from build123d import *

# Parameters (mm, degrees)
F1_DEPTH = 6.35
F2_DEPTH = 6.35
F3_DEPTH = 6.35
F4_DEPTH = 6.35
F5_DEPTH = 6.35


# Not quite as in the source:
# - a feature names something its author has since deleted; it is built from what else it names


with BuildPart() as f1:
    # F0 (on Front) → F1 (new body)
    with BuildSketch(Plane.XZ):
        with BuildLine():
            ThreePointArc((63.0566746496, -7.490379305), (63.3890717721, -3.751743578), (63.5, 0))
            ThreePointArc((63.5, 0), (62.9393473013, 8.4195345051), (61.2672894084, 16.6903939003))
            ThreePointArc((61.2672894084, 16.6903939003), (58.3327446269, 25.0906537239), (54.2527974979, 32.9982418266))
            ThreePointArc((54.2527974979, 32.9982418266), (47.291532101, 42.3764202304), (38.730412603, 50.3210208521))
            ThreePointArc((38.730412603, 50.3210208521), (29.9555685969, 55.9903019284), (20.3699341201, 60.1441250991))
            ThreePointArc((20.3699341201, 60.1441250991), (7.3544916147, 63.0726680353), (-5.9855682874, 63.2172679912))
            ThreePointArc((-5.9855682874, 63.2172679912), (-13.2670335267, 62.09859758), (-20.3699341201, 60.1441250991))
            ThreePointArc((-20.3699341201, 60.1441250991), (-29.9555685969, 55.9903019284), (-38.730412603, 50.3210208521))
            ThreePointArc((-38.730412603, 50.3210208521), (-47.291532101, 42.3764202304), (-54.2527974979, 32.9982418266))
            ThreePointArc((-54.2527974979, 32.9982418266), (-58.3327446269, 25.0906537239), (-61.2672894084, 16.6903939003))
            ThreePointArc((-61.2672894084, 16.6903939003), (-63.3268462658, 4.6862076377), (-63.0566746496, -7.490379305))
            ThreePointArc((-63.0566746496, -7.490379305), (-60.5844983842, -19.0202143924), (-56.023116606, -29.8941533708))
            ThreePointArc((-56.023116606, -29.8941533708), (-49.318773707, -39.9988569841), (-40.8158107072, -48.6448311366))
            ThreePointArc((-40.8158107072, -48.6448311366), (-33.4288158961, -53.9885568226), (-25.3527004473, -58.2193316694))
            ThreePointArc((-25.3527004473, -58.2193316694), (-15.8671551858, -61.4856356095), (-5.9855682874, -63.2172679912))
            ThreePointArc((-5.9855682874, -63.2172679912), (1.1186954333, -63.4901450662), (8.2089360928, -62.9671610304))
            ThreePointArc((8.2089360928, -62.9671610304), (16.9479005402, -61.1965576424), (25.3527004473, -58.2193316694))
            ThreePointArc((25.3527004473, -58.2193316694), (33.4288158961, -53.9885568226), (40.8158107072, -48.6448311366))
            ThreePointArc((40.8158107072, -48.6448311366), (49.318773707, -39.9988569841), (56.023116606, -29.8941533708))
            ThreePointArc((56.023116606, -29.8941533708), (60.5844983842, -19.0202143924), (63.0566746496, -7.490379305))
        make_face()
        with BuildLine():
            ThreePointArc((61.2672894084, 16.6903939003), (62.9393473013, 8.4195345051), (63.5, 0))
            ThreePointArc((63.5, 0), (63.3890717721, -3.751743578), (63.0566746496, -7.490379305))
            Line((63.0566746496, -7.490379305), (88.5324627161, 16.6903939003))
            Line((88.5324627161, 16.6903939003), (61.2672894084, 16.6903939003))
        make_face()
        with BuildLine():
            ThreePointArc((54.2527974979, 32.9982418266), (58.3327446269, 25.0906537239), (61.2672894084, 16.6903939003))
            Line((61.2672894084, 16.6903939003), (71.193754673, 45.4481393099))
            Line((71.193754673, 45.4481393099), (54.2527974979, 32.9982418266))
        make_face()
        with BuildLine():
            Line((85.9054028988, -7.490379305), (63.0566746496, -7.490379305))
            ThreePointArc((63.0566746496, -7.490379305), (60.5844983842, -19.0202143924), (56.023116606, -29.8941533708))
            Line((56.023116606, -29.8941533708), (85.9054028988, -7.490379305))
        make_face()
        with BuildLine():
            ThreePointArc((38.730412603, 50.3210208521), (47.291532101, 42.3764202304), (54.2527974979, 32.9982418266))
            Line((54.2527974979, 32.9982418266), (54.2527974979, 61.2032547377))
            Line((54.2527974979, 61.2032547377), (38.730412603, 50.3210208521))
        make_face()
        with BuildLine():
            ThreePointArc((20.3699341201, 60.1441250991), (29.9555685969, 55.9903019284), (38.730412603, 50.3210208521))
            Line((38.730412603, 50.3210208521), (38.0926132202, 72.2317844629))
            Line((38.0926132202, 72.2317844629), (20.3699341201, 60.1441250991))
        make_face()
        with BuildLine():
            Line((60.1600408554, -63.261911273), (40.8158107072, -48.6448311366))
            ThreePointArc((40.8158107072, -48.6448311366), (33.4288158961, -53.9885568226), (25.3527004473, -58.2193316694))
            Line((25.3527004473, -58.2193316694), (60.1600408554, -63.261911273))
        make_face()
        with BuildLine():
            ThreePointArc((-20.3699341201, 60.1441250991), (-13.2670335267, 62.09859758), (-5.9855682874, 63.2172679912))
            Line((-5.9855682874, 63.2172679912), (-20.3699341201, 81.6848352551))
            Line((-20.3699341201, 81.6848352551), (-20.3699341201, 60.1441250991))
        make_face()
        with BuildLine():
            ThreePointArc((-38.730412603, 50.3210208521), (-29.9555685969, 55.9903019284), (-20.3699341201, 60.1441250991))
            Line((-20.3699341201, 60.1441250991), (-38.0926132202, 72.2317844629))
            Line((-38.0926132202, 72.2317844629), (-38.730412603, 50.3210208521))
        make_face()
        with BuildLine():
            ThreePointArc((-54.2527974979, 32.9982418266), (-47.291532101, 42.3764202304), (-38.730412603, 50.3210208521))
            Line((-38.730412603, 50.3210208521), (-54.2527974979, 61.2032547377))
            Line((-54.2527974979, 61.2032547377), (-54.2527974979, 32.9982418266))
        make_face()
        with BuildLine():
            Line((-60.1600408554, -63.261911273), (-25.3527004473, -58.2193316694))
            ThreePointArc((-25.3527004473, -58.2193316694), (-33.4288158961, -53.9885568226), (-40.8158107072, -48.6448311366))
            Line((-40.8158107072, -48.6448311366), (-60.1600408554, -63.261911273))
        make_face()
        with BuildLine():
            ThreePointArc((-61.2672894084, 16.6903939003), (-58.3327446269, 25.0906537239), (-54.2527974979, 32.9982418266))
            Line((-54.2527974979, 32.9982418266), (-71.193754673, 45.4481393099))
            Line((-71.193754673, 45.4481393099), (-61.2672894084, 16.6903939003))
        make_face()
        with BuildLine():
            ThreePointArc((-63.0566746496, -7.490379305), (-63.3268462658, 4.6862076377), (-61.2672894084, 16.6903939003))
            Line((-61.2672894084, 16.6903939003), (-88.5324627161, 16.6903939003))
            Line((-88.5324627161, 16.6903939003), (-63.0566746496, -7.490379305))
        make_face()
        with BuildLine():
            Line((-85.9054028988, -7.490379305), (-56.023116606, -29.8941533708))
            ThreePointArc((-56.023116606, -29.8941533708), (-60.5844983842, -19.0202143924), (-63.0566746496, -7.490379305))
            Line((-63.0566746496, -7.490379305), (-85.9054028988, -7.490379305))
        make_face()
    extrude(amount=F1_DEPTH)

    # F0 (on Front) → F2 (join)
    with BuildSketch(Plane.XZ):
        with BuildLine():
            Line((-73.2954144478, -38.053765893), (-40.8158107072, -48.6448311366))
            ThreePointArc((-40.8158107072, -48.6448311366), (-49.318773707, -39.9988569841), (-56.023116606, -29.8941533708))
            Line((-56.023116606, -29.8941533708), (-73.2954144478, -38.053765893))
        make_face()
        with BuildLine():
            Line((73.2954144478, -38.053765893), (56.023116606, -29.8941533708))
            ThreePointArc((56.023116606, -29.8941533708), (49.318773707, -39.9988569841), (40.8158107072, -48.6448311366))
            Line((40.8158107072, -48.6448311366), (73.2954144478, -38.053765893))
        make_face()
    extrude(amount=F2_DEPTH)

    # F0 (on Front) → F3 (join)
    with BuildSketch(Plane.XZ):
        with BuildLine():
            Line((0, -92.2421216965), (8.2089360928, -62.9671610304))
            ThreePointArc((8.2089360928, -62.9671610304), (1.1186954333, -63.4901450662), (-5.9855682874, -63.2172679912))
            Line((-5.9855682874, -63.2172679912), (0, -92.2421216965))
        make_face()
        with BuildLine():
            ThreePointArc((-5.9855682874, 63.2172679912), (7.3544916147, 63.0726680353), (20.3699341201, 60.1441250991))
            Line((20.3699341201, 60.1441250991), (0, 92.2421216965))
            Line((0, 92.2421216965), (-5.9855682874, 63.2172679912))
        make_face()
    extrude(amount=F3_DEPTH)

    # F0 (on Front) → F4 (join)
    with BuildSketch(Plane.XZ):
        with BuildLine():
            Line((-20.3699341201, -81.6848352551), (-5.9855682874, -63.2172679912))
            ThreePointArc((-5.9855682874, -63.2172679912), (-15.8671551858, -61.4856356095), (-25.3527004473, -58.2193316694))
            Line((-25.3527004473, -58.2193316694), (-20.3699341201, -81.6848352551))
        make_face()
        with BuildLine():
            Line((60.1600408554, -63.261911273), (40.8158107072, -48.6448311366))
            ThreePointArc((40.8158107072, -48.6448311366), (33.4288158961, -53.9885568226), (25.3527004473, -58.2193316694))
            Line((25.3527004473, -58.2193316694), (60.1600408554, -63.261911273))
        make_face()
    extrude(amount=F4_DEPTH)

    # F0 (on Front) → F5 (join)
    with BuildSketch(Plane.XZ):
        with BuildLine():
            Line((22.25664258, -86.1358046532), (25.3527004473, -58.2193316694))
            ThreePointArc((25.3527004473, -58.2193316694), (16.9479005402, -61.1965576424), (8.2089360928, -62.9671610304))
            Line((8.2089360928, -62.9671610304), (22.25664258, -86.1358046532))
        make_face()
    extrude(amount=F5_DEPTH)


solid = f1.part
Geometry check sheet. Reference: the model listing, model coordinates, mm. A direction names the side the tool comes from. Give positions to 0.01 mm unless a question says otherwise; leave off trailing zeros. Order: outer loops, then holes, each group sorted by start corner. A loop starts at its lowest first (then second) coordinate and runs counter-clockwise, first axis right, second up. Notation, with made-up numbers: M -3.75,-29 L 7.25,-29 A28 cw 7.25,9 Z; hole C -25,66.5 d7. An arc over 180 degrees is marked long. Use a Markdown table: item, result.
Item 1: Draft check along Z on faces 5 (the flat face through (42.513, -3.131, -60.705)), 6 (the flat face through (-2.95, -3.13, 77.93)), 7 (the flat face through (-50.35, -3.13, -55.85)). Enter one of: +Z half, -Z half, draft (parallel to the pull), parting line (faces both ways), or undercut.
Answers follow:
| item | result |
|---|---|
| face 5 | -Z half |
| face 6 | +Z half |
| face 7 | undercut |
Item 2: Section check D-D (x = -48). Record the cut outline in (y, z), and give its area (3 significant figures).
Answers follow:
| item | result |
|---|---|
| outline | M -6.35,-61.5 L 0,-61.5 L 0,-54.07 L -6.35,-54.07 Z; M -6.35,-46.3 L 0,-46.3 L 0,56.82 L -6.35,56.82 Z |
| area | 702 mm2 |
Item 3: Section check B-B (x = -66). Record the cut outline in (y, z), and give its area (3 significant figures).
Answers follow:
| item | result |
|---|---|
| outline | M -6.35,-40.43 L 0,-40.43 L 0,-34.61 L -6.35,-34.61 Z; M -6.35,-22.41 L 0,-22.41 L 0,-7.49 L -6.35,-7.49 Z; M -6.35,-4.7 L 0,-4.7 L 0,16.69 L -6.35,16.69 Z; M -6.35,30.4 L 0,30.4 L 0,41.63 L -6.35,41.63 Z |
| area | 339 mm2 |
Item 4: Section check A-A (z = 53). Record the cut outline in (x, y), and give its area (3 significant figures).
Answers follow:
| item | result |
|---|---|
| outline | M -54.25,-6.35 L -42.55,-6.35 L -42.55,0 L -54.25,0 Z; M -38.65,-6.35 L 38.65,-6.35 L 38.65,0 L -38.65,0 Z; M 42.55,-6.35 L 54.25,-6.35 L 54.25,0 L 42.55,0 Z |
| area | 639 mm2 |
Item 5: Material ranges on line 1 along X through (y, z) = (-5.75, -79); line 2 along X through (y, z) = (-3, 63); line 3 along X through (y, z) = (-0.25, 68.5), recorded low to high.
Answers follow:
| item | result |
|---|---|
| line 1 | x = -20.94 to -18.28, -2.73 to 3.71, 17.93 to 23.05 |
| line 2 | x = -38.36 to -24.56, -20.37 to 18.56, 24.56 to 38.36 |
| line 3 | x = -38.2 to -32.62, -20.37 to -10.1, -4.9 to 15.07, 32.62 to 38.2 |
Item 6: Tool access check on faces 1 (the flat face through (-75.973, -3.131, 4.769)), 2 (the flat face through (-13.28, -3.13, -72.58)), 3 (the flat face through (62.84, -3.13, 39.31)), 4 (the flat face through (75, -3, 16.69)). Record the directions out of +Z, -Z, +X, -X, +Y, -Y that give a thin tool (end or side, any length) a straight path to the whole face; none if there is none.
Answers follow:
| item | result |
|---|---|
| face 1 | -X, +Y, -Y |
| face 2 | -Z, +Y, -Y |
| face 3 | +Z, +Y, -Y |
| face 4 | +X, +Y, -Y |
Item 7: Section check C-C (x = 50). Record the cut outline in (y, z).
Answers follow:
| item | result |
|---|---|
| outline | M -6.35,-61.79 L 0,-61.79 L 0,-55.58 L -6.35,-55.58 Z; M -6.35,-45.65 L 0,-45.65 L 0,58.22 L -6.35,58.22 Z |
Item 8: Depth check by flat-ended pin: P1, Ø1.5, axis at x = -66.5, z = 25.5, coming from the +Y side; P2, Ø2, axis at x = 7, y = -3.5, coming from the +Z side; P3, Ø3, axis at x = 72.5, y = -2, coming from the +Z side; P4, Ø1, axis at x = 47.5, z = -22.5, coming from the +Y side. Enter the tip coordinate at first touch or a pass-through.
Answers follow:
| item | result |
|---|---|
| P1 | passes through |
| P2 | stops at z = 82.79 |
| P3 | stops at z = 45.45 |
| P4 | stops at y = 0 |
